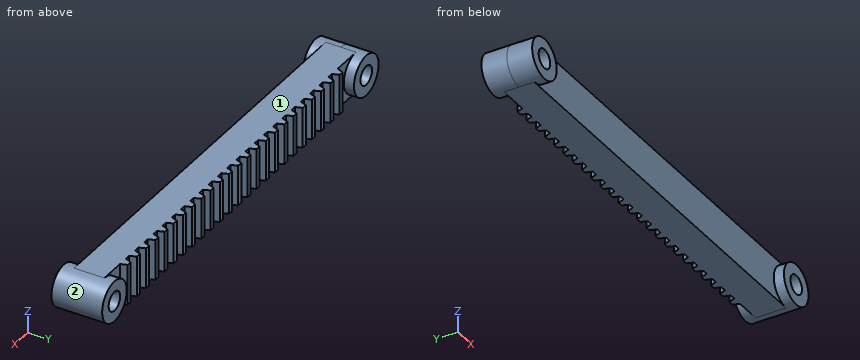
from build123d import *

# Parameters (mm, degrees)
BOSS_EXTRUDE1_DEPTH = 6
SKETCH1_3_R         = 8
SKETCH1_3_R_2       = 3.75
BOSS_EXTRUDE2_DEPTH = 10
BOSS_EXTRUDE3_DEPTH = 16


with BuildPart() as part:
    # Sketch1 → Boss-Extrude1 (new body, symmetric)
    with BuildSketch(Plane(origin=(0, 0, 0), x_dir=(1, 0, 0), z_dir=(0, 1, 0))):
        with BuildLine():
            Line((82, 8), (-82, 8))
            ThreePointArc((-82, 8), (-76.343145751, 5.656854249), (-74, 0))
            ThreePointArc((-74, 0), (-76.343145751, -5.656854249), (-82, -8))
            Line((-82, -8), (82, -8))
            ThreePointArc((82, -8), (74, 0), (82, 8))
        make_face()
    extrude(amount=BOSS_EXTRUDE1_DEPTH, both=True)

    # Sketch1_3 → Boss-Extrude2 (add, symmetric)
    with BuildSketch(Plane(origin=(0, 0, 0), x_dir=(1, 0, 0), z_dir=(0, 1, 0))):
        with Locations((-82, 0)):
            Circle(SKETCH1_3_R)
        with Locations((-82, 0)):
            Circle(SKETCH1_3_R_2, mode=Mode.SUBTRACT)
        with Locations((82, 0)):
            Circle(SKETCH1_3_R)
        with Locations((82, 0)):
            Circle(SKETCH1_3_R_2, mode=Mode.SUBTRACT)
    extrude(amount=BOSS_EXTRUDE2_DEPTH, both=True)

    # Sketch2 → Boss-Extrude3 (add)
    with BuildSketch(Plane.XY.offset(8)):
        Polygon((71.819851171, 6), (70.909925586, 8.5), (68.909925586, 8.5), (68, 6), align=None)
        Polygon((65.819851171, 6), (64.909925586, 8.5), (62.909925586, 8.5), (62, 6), align=None)
        Polygon((59.819851171, 6), (58.909925586, 8.5), (56.909925586, 8.5), (56, 6), align=None)
        Polygon((53.819851171, 6), (52.909925586, 8.5), (50.909925586, 8.5), (50, 6), align=None)
        Polygon((47.819851171, 6), (46.909925586, 8.5), (44.909925586, 8.5), (44, 6), align=None)
        Polygon((41.819851171, 6), (40.909925586, 8.5), (38.909925586, 8.5), (38, 6), align=None)
        Polygon((35.819851171, 6), (34.909925586, 8.5), (32.909925586, 8.5), (32, 6), align=None)
        Polygon((29.819851171, 6), (28.909925586, 8.5), (26.909925586, 8.5), (26, 6), align=None)
        Polygon((23.819851171, 6), (22.909925586, 8.5), (20.909925586, 8.5), (20, 6), align=None)
        Polygon((17.819851171, 6), (16.909925586, 8.5), (14.909925586, 8.5), (14, 6), align=None)
        Polygon((11.819851171, 6), (10.909925586, 8.5), (8.909925586, 8.5), (8, 6), align=None)
        Polygon((5.819851171, 6), (4.909925586, 8.5), (2.909925586, 8.5), (2, 6), align=None)
        Polygon((-0.180148829, 6), (-1.090074414, 8.5), (-3.090074414, 8.5), (-4, 6), align=None)
        Polygon((-6.180148829, 6), (-7.090074414, 8.5), (-9.090074414, 8.5), (-10, 6), align=None)
        Polygon((-12.180148829, 6), (-13.090074414, 8.5), (-15.090074414, 8.5), (-16, 6), align=None)
        Polygon((-18.180148829, 6), (-19.090074414, 8.5), (-21.090074414, 8.5), (-22, 6), align=None)
        Polygon((-24.180148829, 6), (-25.090074414, 8.5), (-27.090074414, 8.5), (-28, 6), align=None)
        Polygon((-30.180148829, 6), (-31.090074414, 8.5), (-33.090074414, 8.5), (-34, 6), align=None)
        Polygon((-36.180148829, 6), (-37.090074414, 8.5), (-39.090074414, 8.5), (-40, 6), align=None)
        Polygon((-42.180148829, 6), (-43.090074414, 8.5), (-45.090074414, 8.5), (-46, 6), align=None)
        Polygon((-48.180148829, 6), (-49.090074414, 8.5), (-51.090074414, 8.5), (-52, 6), align=None)
        Polygon((-54.180148829, 6), (-55.090074414, 8.5), (-57.090074414, 8.5), (-58, 6), align=None)
        Polygon((-60.180148829, 6), (-61.090074414, 8.5), (-63.090074414, 8.5), (-64, 6), align=None)
        Polygon((-66.180148829, 6), (-67.090074414, 8.5), (-69.090074414, 8.5), (-70, 6), align=None)
    extrude(amount=-BOSS_EXTRUDE3_DEPTH)


solid = part.part
For this review, take the finished solid that the model builds, in its own axes (mm). Face numbers are marked on the shaded views. Round coordinates to 2 decimals unless told otherwise and drop trailing zeros. Order: outer loops, then holes, each group sorted by start corner. A loop starts at its lowest first (then second) coordinate and runs counter-clockwise, first axis right, second up. Notation, with made-up numbers: (64, 79.25) -> (110, 79.25) arc R23 ccw to (110, 116.25) -> close; hole circle Ø9 at (-18, 77.25). An arc over 180 degrees is marked (long way). Put each result on its own line as item: value.
Q1. Add section B-B on z = 0. State how many separate pieces and enclosed holes the cut face has, plus the area to 3 significant figures.
Check result:
separate pieces: 3
enclosed holes: 0
area: 2,290 mm2
Q2. Insertion check: pin 1 Ø1.6 at (x, z) = (16, 1) entering from +Y; pin 2 Ø1.5 at (x, z) = (-62, -5) entering from -Y; pin 3 Ø2 at (y, z) = (-3.5, -2) entering from -X. Each pin has a flat end and moves straight along its axis. Give the tip position at first contact, or say it passes through.
Check result:
pin 1: y = 8.5
pin 2: y = -6
pin 3: x = -89.94
Q3. Add section C-C on y = 1.5. Write out the cut boundary in (x, z), plus the area to 3 significant figures.
Check result:
outline: (-82, -8) -> (82, -8) arc R8 ccw to (82, 8) -> (-82, 8) arc R8 ccw to start; hole circle Ø7.5 at (-82, 0); hole circle Ø7.5 at (82, 0)
area: 2,740 mm2
Q4. Mouldability with a two-part tool opening along X and no side actions: class the marked faces 1 and 2 as pulls with the +X half, pulls with the -X half, needs draft (parallel to the pull), parting line crosses it, or undercut.
Check result:
face 1: needs draft
face 2: undercut
Q5. For probe 1 along X at (y, z) = (3.5, 0); probe 2 along X at (y, z) = (-7, 0); probe 3 along Z at (x, y) = (-82, 8.25), list the stretches that pass through material, from the lowest coordinate up. Write a range as [from, to].
Check result:
probe 1: [-90, -85.75], [-78.25, 78.25], [85.75, 90]
probe 2: [-90, -85.75], [-78.25, -74], [74, 78.25], [85.75, 90]
probe 3: [-8, -3.75], [3.75, 8]
Q6. Add section A-A on y = -7.5. Write out the cut boundary in (x, z), plus the area to 3 significant figures.
Check result:
outline: circle Ø16 at (-82, 0); circle Ø16 at (82, 0); hole circle Ø7.5 at (-82, 0); hole circle Ø7.5 at (82, 0)
area: 314 mm2
